Part model, mm, in its own coordinate system. A direction names the side the tool comes from. Coordinates: 2 decimals unless noted, no trailing zeros. Loops run counter-clockwise (first coordinate to the right, second up) from the corner with the lowest first, then second, coordinate; pieces in that order, holes last. Notation, with made-up numbers: (83, 82.5) -> (137, 82.5) arc R16 cw to (137, 112.5) -> close; hole circle Ø4 at (-35, 40). An arc over 180 degrees is marked (long way). One line per question, with ' | ' between items. Start each with the question number.
1) Probe L1, parallel to Y at x = 3.25, z = 2.75 (3 decimals); L2, parallel to X at y = 23.5, z = -2.75; L3, parallel to X at y = 10.75, z = -1.25. List the from-to ranges inside material, lowest first. Write a range as from..to.
2) 3-axis set-ups, long thin cutter, end or side, ignore diameter. For faces 1 (the face through (-4, 20.955, 0)), 2 (the face through (0, 25.4, 0)): which of +Z, -Z, +X, -X, +Y, -Y reach the whole face in a straight line?
3) Drop a flat-ended pin along its axis: pin 1 (3 mm diameter, centred on x = -1, z = 0.5, fed in from -Y). Give the stop position or say it passes through.
4) Cut at A-A (x = 0). List the corners of the cut face in (y, z) (1 decimal).
5) Cut at B-B (z = 0). List the corners of the cut face in (x, y) (1 decimal), plus the area to 3 significant figures.
6) Cut at D-D (y = 8). List the corners of the cut face in (x, z) (1 decimal).
7) Cut at C-C (z = -4). List the corners of the cut face in (x, y) (3 decimals), plus the area to 3 significant figures.
8) Two-plate mould, pull along Y, no slides. Class faces 3 (the face through (-2.9, 24.11, -3.78)), 4 (the face through (-3.463, 21.921, -0.455)), 5 (the face through (0, 0, 0)): released by +Y, released by -Y, zero draft, split by the parting line, or undercut.
from build123d import *

# Parameters (mm, degrees)
SKETCH1_R           = 4.7625
BOSS_EXTRUDE1_DEPTH = 25.4
SKETCH2_W           = 2.54
SKETCH2_H           = 1.905


with BuildPart() as part:
    # Sketch1 → Boss-Extrude1 (new body)
    with BuildSketch(Plane(origin=(0, 0, 0), x_dir=(1, 0, 0), z_dir=(0, 1, 0))):
        with Locations(Location((0, 0, 0), (0, 0, 270))):
            Circle(SKETCH1_R)
    extrude(amount=BOSS_EXTRUDE1_DEPTH)

    # Sketch2 → Cut-Revolve1 (revolve, cut)
    with BuildSketch(Plane(origin=(0, 0, 0), x_dir=(0, 0, -1), z_dir=(1, 0, 0)), mode=Mode.PRIVATE) as cut_revolve1_sk:
        with Locations((4.7625, 21.9075)):
            Rectangle(SKETCH2_W, SKETCH2_H)
        with Locations((4.7625, 16.1925)):
            Rectangle(SKETCH2_W, SKETCH2_H)
    revolve(cut_revolve1_sk.sketch.rotate(Axis((0, 25.4, 0), (0, -1, 0)), 180), axis=Axis((0, 25.4, 0), (0, -1, 0)), mode=Mode.SUBTRACT)


solid = part.part
Reported:
1) L1: y = 0..15.24, 17.145..20.955, 22.86..25.4 | L2: x = -3.89..3.89 | L3: x = -4.6..4.6
2) face 1: none | face 2: +Z, -Z, +X, -X, +Y
3) pin 1: stops at y = 0
4) outline: (0, -4.8) -> (15.2, -4.8) -> (15.2, -3.5) -> (17.1, -3.5) -> (17.1, -4.8) -> (21, -4.8) -> (21, -3.5) -> (22.9, -3.5) -> (22.9, -4.8) -> (25.4, -4.8) -> (25.4, 4.8) -> (22.9, 4.8) -> (22.9, 3.5) -> (21, 3.5) -> (21, 4.8) -> (17.1, 4.8) -> (17.1, 3.5) -> (15.2, 3.5) -> (15.2, 4.8) -> (0, 4.8) -> close
5) outline: (-4.8, 0) -> (4.8, 0) -> (4.8, 15.2) -> (3.5, 15.2) -> (3.5, 17.1) -> (4.8, 17.1) -> (4.8, 21) -> (3.5, 21) -> (3.5, 22.9) -> (4.8, 22.9) -> (4.8, 25.4) -> (-4.8, 25.4) -> (-4.8, 22.9) -> (-3.5, 22.9) -> (-3.5, 21) -> (-4.8, 21) -> (-4.8, 17.1) -> (-3.5, 17.1) -> (-3.5, 15.2) -> (-4.8, 15.2) -> close | area: 232 mm²
6) outline: circle Ø9.5 at (0, 0)
7) outline: (-2.585, 0) -> (2.585, 0) -> (2.585, 15.24) -> (-2.585, 15.24) -> close; (-2.585, 17.145) -> (2.585, 17.145) -> (2.585, 20.955) -> (-2.585, 20.955) -> close; (-2.585, 22.86) -> (2.585, 22.86) -> (2.585, 25.4) -> (-2.585, 25.4) -> close | area: 112 mm²
8) face 3: zero draft | face 4: undercut | face 5: released by -Y
